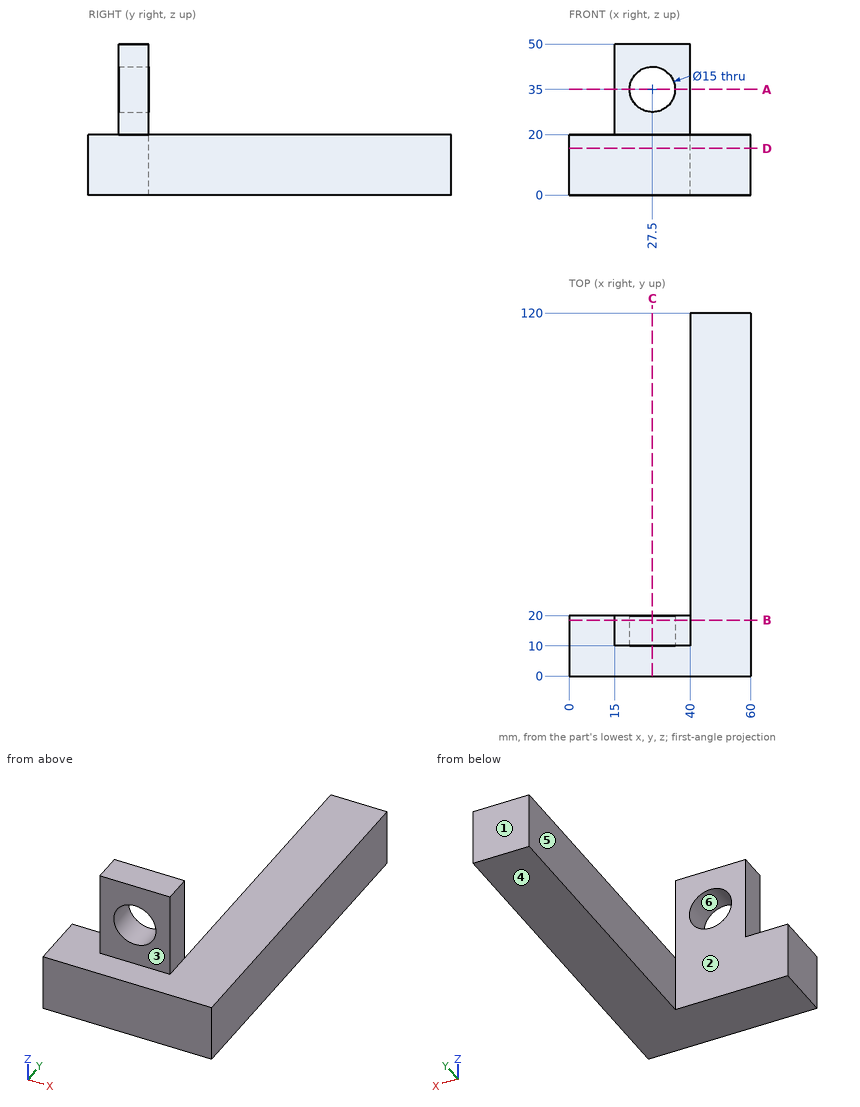
Check sheet for the drawn part. Datum: minimum x, y, z corner. Units: mm. A direction names the side the tool comes from. Round coordinates to 2 decimals unless told otherwise and drop trailing zeros. Write each loop counter-clockwise with the first axis right and the second up, starting at its lowest first coordinate (ties: lowest second). Pieces come first, ordered by that corner, then holes. Notation, with made-up numbers: (7, 67.5) -> (55, 67.5) arc R22 cw to (55, 105.5) -> close; hole circle Ø8 at (31.5, -17.5). An arc over 180 degrees is marked (long way). Write each question's results on one line, items separated by ' | '.
Q1. Sectioned sample at B-B, the plane y = 18.5. Record the boundary of the cut face in (x, z), and give its area (3 significant figures).
Derived:
outline: (0, 0) -> (60, 0) -> (60, 20) -> (40, 20) -> (40, 50) -> (15, 50) -> (15, 20) -> (0, 20) -> close; hole circle Ø15 at (27.5, 35) | area: 1,770 mm²
Q2. Sectioned sample at C-C, the plane x = 27.5. Record the boundary of the cut face in (y, z).
Derived:
outline: (0, 0) -> (20, 0) -> (20, 27.5) -> (10, 27.5) -> (10, 20) -> (0, 20) -> close; (10, 42.5) -> (20, 42.5) -> (20, 50) -> (10, 50) -> close
Q3. Access from +Z, -Z, +X, -X, +Y, -Y to the whole of each face (thin tool, end or side, straight path). Record for the marked faces 1, 2 and 3.
Derived:
face 1: +Z, -Z, +X, -X, +Y | face 2: +Z, -Z, -X, +Y | face 3: +Z, +X, -X, -Y
Q4. Sectioned sample at A-A, the plane z = 35. Record the boundary of the cut face in (x, y), and give its area (3 significant figures).
Derived:
outline: (15, 10) -> (20, 10) -> (20, 20) -> (15, 20) -> close; (35, 10) -> (40, 10) -> (40, 20) -> (35, 20) -> close | area: 100 mm²
Q5. Draft check along Z on the marked faces 4, 5 and 6. Enter one of: released by +Z, released by -Z, zero draft, split by the parting line, or undercut.
Derived:
face 4: released by -Z | face 5: zero draft | face 6: undercut
Q6. Sectioned sample at D-D, the plane z = 15.5. Record the boundary of the cut face in (x, y).
Derived:
outline: (0, 0) -> (60, 0) -> (60, 120) -> (40, 120) -> (40, 20) -> (0, 20) -> close
Q7. Thickness scan on probe 1 along Z at (x, y) = (27, 18); probe 2 along X at (y, z) = (11.5, 34.5); probe 3 along Z at (x, y) = (48.5, 65). Record the ranges inside material, lowest first.
Derived:
probe 1: z = 0 to 27.52, 42.48 to 50 | probe 2: x = 15 to 20.02, 34.98 to 40 | probe 3: z = 0 to 20
Q8. Go/stop test with flat-tipped pins: pin 1 Ø5 at (x, y) = (49.5, 59) entering from +Z; pin 2 Ø20 at (x, z) = (13, 31.5) entering from +Y; pin 3 Ø10 at (y, z) = (65.5, 12) entering from -X; pin 4 Ø12 at (x, z) = (53, 27.5) entering from -Y. Record where each tip stops, or that it passes through.
Derived:
pin 1: stops at z = 20 | pin 2: stops at y = 20 | pin 3: stops at x = 40 | pin 4: passes through
